from build123d import *

# Parameters (mm, degrees)
SKETCH1_W                  = 3.95
SKETCH1_H                  = 13.1
BOSS_EXTRUDE1_DEPTH        = 13
SKETCH2_W                  = 3.95
SKETCH2_H                  = 13.1
BOSS_EXTRUDE2_DEPTH        = 13
BOSS_EXTRUDE3_REACH        = 37.222
SKETCH3_W                  = 6.25
SKETCH3_H                  = 7
SKETCH10_W                 = 8.025
SKETCH10_H                 = 7
BOSS_EXTRUDE7_DEPTH        = 6.25
FILLET7_R                  = 1
SKETCH11_W                 = 33.95
SKETCH11_H                 = 6.25
BOSS_EXTRUDE8_DEPTH        = 30.5283
F_3_2_3_2_DIAMETER_HOLE1_D = 3.2
FILLET8_START              = -7
FILLET8_DEPTH              = 8
FILLET8_START_2            = -6.25
FILLET8_2_DEPTH            = 6.25
FILLET9_R                  = 1


with BuildPart() as part:
    # Sketch1 → Boss-Extrude1 (new body)
    with BuildSketch(Plane(origin=(0, 0, 0), x_dir=(1, 0, 0), z_dir=(0, 1, 0))):
        with Locations((0, 6.55)):
            Rectangle(SKETCH1_W, SKETCH1_H)
    extrude(amount=BOSS_EXTRUDE1_DEPTH)


with BuildPart() as body_2:
    # Sketch2 → Boss-Extrude2 (new body)
    with BuildSketch(Plane(origin=(0, 0, 0), x_dir=(1, 0, 0), z_dir=(0, 1, 0))):
        with Locations((30, 6.55)):
            Rectangle(SKETCH2_W, SKETCH2_H)
    extrude(amount=BOSS_EXTRUDE2_DEPTH)

    # Sketch3 → Boss-Extrude3 (add, up to next)
    with BuildSketch(Plane(origin=(1.975, 0, 0), x_dir=(0, 0, -1), z_dir=(1, 0, 0)), mode=Mode.PRIVATE) as boss_extrude3_sk1:
        with Locations((3.125, 9.5)):
            Rectangle(SKETCH3_W, SKETCH3_H)
    boss_extrude3_tool1 = extrude(boss_extrude3_sk1.sketch, amount=BOSS_EXTRUDE3_REACH, mode=Mode.PRIVATE) - body_2.part

    add(part.part)  # Boss-Extrude3 merges part
    add(boss_extrude3_tool1.solids().sort_by_distance((1.975, 9.5, -3.125))[0])

    # Sketch10 → Boss-Extrude7 (add)
    with BuildSketch(Plane.XY):
        with Locations((-5.9875, 9.5)):
            Rectangle(SKETCH10_W, SKETCH10_H)
        with Locations((35.9875, 9.5)):
            Rectangle(SKETCH10_W, SKETCH10_H)
    extrude(amount=-BOSS_EXTRUDE7_DEPTH)

    # Fillet7
    fillet7_edges = [body_2.edges().sort_by_distance(p)[0] for p in [
        (28.025, 0, -6.55),
        (31.975, 0, -6.55),
        (1.975, 0, -6.55),
        (-1.975, 0, -6.55),
    ]]
    fillet(fillet7_edges, radius=FILLET7_R)

    # Sketch11 → Boss-Extrude8 (add)
    with BuildSketch(Plane(origin=(0, 13, 0), x_dir=(1, 0, 0), z_dir=(0, 1, 0))):
        with Locations((15, 3.125)):
            Rectangle(SKETCH11_W, SKETCH11_H)
    extrude(amount=BOSS_EXTRUDE8_DEPTH)

    # Ø3.2 (3.2) Diameter Hole1 (through all)
    with Locations(Plane.XY):
        with Locations((28.025, 40.3533), (1.975, 40.3533)):
            Hole(F_3_2_3_2_DIAMETER_HOLE1_D / 2)

    # Fillet8: read off the stored shape, not the designer's step
    # Fillet8 outline → Fillet8 (cut)
    with BuildSketch(Plane.XY.offset(FILLET8_START)):
        with BuildLine():
            Line((40, 13), (37.5, 13))
            ThreePointArc((37.5, 13), (39.267766953, 12.267766953), (40, 10.5))
            Line((40, 10.5), (40, 13))
        make_face()
        with BuildLine():
            Line((-10, 13), (-10, 10.5))
            ThreePointArc((-10, 10.5), (-9.267766953, 12.267766953), (-7.5, 13))
            Line((-7.5, 13), (-10, 13))
        make_face()
    extrude(amount=FILLET8_DEPTH, mode=Mode.SUBTRACT)

    # Fillet8 2 outline → Fillet8 2 (add)
    with BuildSketch(Plane.XY.offset(FILLET8_START_2)):
        with BuildLine():
            Line((31.975, 13), (34.475, 13))
            ThreePointArc((34.475, 13), (32.707233047, 13.732233047), (31.975, 15.5))
            Line((31.975, 15.5), (31.975, 13))
        make_face()
        with BuildLine():
            ThreePointArc((-1.975, 15.5), (-2.707233047, 13.732233047), (-4.475, 13))
            Line((-4.475, 13), (-1.975, 13))
            Line((-1.975, 13), (-1.975, 15.5))
        make_face()
    extrude(amount=FILLET8_2_DEPTH)

    # Fillet9
    fillet9_edges = [body_2.edges().sort_by_distance(p)[0] for p in [
        (28.025, 6, -3.125),
        (1.975, 6, -3.125),
        (-1.975, 6, -3.125),
        (31.975, 6, -3.125),
    ]]
    fillet(fillet9_edges, radius=FILLET9_R)


solid = body_2.part
Geometry: final body of the model. Coordinates: model frame, mm. A direction names the side the tool comes from. Round coordinates to 2 decimals unless told otherwise and drop trailing zeros. Order: outer loops, then holes, each group sorted by start corner. A loop starts at its lowest first (then second) coordinate and runs counter-clockwise, first axis right, second up. Notation, with made-up numbers: (89.5, -16.75) - (115.5, -16.75) arc R14 ccw to (115.5, -2.75) - close; hole circle Ø9 at (-17.5, 37). An arc over 180 degrees is marked (long way). Write each question's results on one line, items separated by ' | '.
Item 1: Mould query, pull axis Y, two halves, no side actions, for faces 1 (the flat face through (31.975, 6, -8)), 2 (the cylindrical face through (29.295, 39.38, -3.169)), 3 (the flat face through (15, 6, -3)). Classes: pulls with the +Y half, pulls with the -Y half, needs draft (parallel to the pull), parting line crosses it, or undercut.
Completed:
face 1: needs draft | face 2: undercut | face 3: pulls with the -Y half
Item 2: Section A-A, the plane z = -11.75. Return the cut outline in (x, y) (3 decimals).
Completed:
outline: (-1.975, 1) arc R1 ccw to (-0.975, 0) - (0.975, 0) arc R1 ccw to (1.975, 1) - (1.975, 13) - (-1.975, 13) - close; (28.025, 1) arc R1 ccw to (29.025, 0) - (30.975, 0) arc R1 ccw to (31.975, 1) - (31.975, 13) - (28.025, 13) - close
Item 3: Reachability of faces 4 (the flat face through (-6, 13, -3)), 5 (the flat face through (28.025, 6, -8)), 6 (the flat face through (36, 13, -3)), 7 (the flat face through (-1.975, 6, -8)) from +Z, -Z, +X, -X, +Y, -Y: full face, straight path, thin tool, end or side. Return the list, or none.
Completed:
face 4: +Z, -Z, -X, +Y | face 5: -Z, -Y | face 6: +Z, -Z, +X, +Y | face 7: -Z, -X, -Y
Item 4: Material intervals for line 1 along X through (y, z) = (12.5, -6.5) (3 decimals); line 2 along Z through (x, y) = (6.5, 7); line 3 along X through (y, z) = (41, -1.5) (3 decimals), sorted ascending. Write a range as [from, to].
Completed:
line 1: [-1.975, 1.975], [28.025, 31.975] | line 2: [-6.25, 0] | line 3: [-1.975, 0.512], [3.438, 26.562], [29.488, 31.975]
Item 5: Section D-D, the plane x = 4.5. Return the cut outline in (y, z).
Completed:
outline: (6, -6.25) - (43.53, -6.25) - (43.53, 0) - (6, 0) - close
Item 6: Section C-C, the plane y = 29. Return the cut outline in (x, z) (3 decimals), and give its area (3 significant figures).
Completed:
outline: (-1.975, -6.25) - (31.975, -6.25) - (31.975, 0) - (-1.975, 0) - close | area: 212 mm^2
Item 7: First-contact query: pin 1 Ø2 at (x, z) = (-0.5, -8) entering from +Y; pin 2 Ø5 at (x, y) = (1.98, 40.35) entering from -Z; pin 3 Ø7 at (y, z) = (22.5, -1.5) entering from -X (3 decimals). Flat tips, straight axial feed; report the tip coordinate or a pass-through.
Completed:
pin 1: y = 13 | pin 2: z = -6.25 | pin 3: x = -1.975
Item 8: Section B-B, the plane z = -3.5. State how many separate pieces and enclosed holes the cut face has, and give its area (3 significant figures).
Completed:
separate pieces: 1 | enclosed holes: 2 | area: 1,420 mm^2
